```python
from build123d import *

# Parameters (mm, degrees)
EXTRUDE_1_DEPTH     = 24
SKETCH_2_R          = 1.6
CUT_EXTRUDE_1_DEPTH = 6.8
SKETCH_3_R          = 3.15
CUT_EXTRUDE_2_DEPTH = 26.4


with BuildPart() as part:
    # 草圖1 → 填料-伸長1 (new body, symmetric)
    with BuildSketch(Plane.XY):
        Polygon((0, 0), (0, 33), (26.4, 33), (26.4, 0), (22.4, 0), (22.4, 27.2), (4, 27.2), (4, 0), align=None)
    extrude(amount=EXTRUDE_1_DEPTH, both=True)

    # 草圖2 → 除料-伸長1 (cut, through all)
    with BuildSketch(Plane.XZ.offset(-27.2)):
        with Locations((7.719922446, 5.480077554)):
            Circle(SKETCH_2_R)
        with Locations((18.680077554, 5.480077554)):
            Circle(SKETCH_2_R)
        with Locations((18.680077554, -5.480077554)):
            Circle(SKETCH_2_R)
        with Locations((7.719922446, -5.480077554)):
            Circle(SKETCH_2_R)
    extrude(amount=-CUT_EXTRUDE_1_DEPTH, mode=Mode.SUBTRACT)

    # 草圖3 → 除料-伸長2 (cut)
    with BuildSketch(Plane(origin=(26.4, 0, 0), x_dir=(0, 0, -1), z_dir=(1, 0, 0))):
        with Locations((0, 6)):
            Circle(SKETCH_3_R)
        with Locations((15, 6)):
            Circle(SKETCH_3_R)
        with Locations((-15, 6)):
            Circle(SKETCH_3_R)
    extrude(amount=-CUT_EXTRUDE_2_DEPTH, mode=Mode.SUBTRACT)


solid = part.part
```
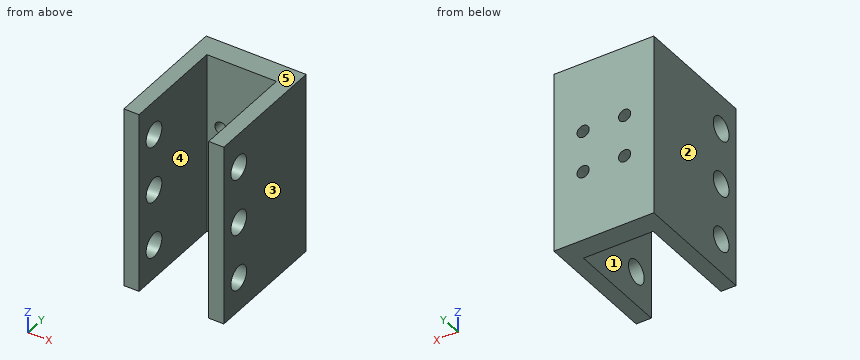
For this review, take the finished solid that the model builds, in its own axes (mm). Face numbers are marked on the shaded views. A direction names the side the tool comes from. Round coordinates to 2 decimals unless told otherwise and drop trailing zeros. Write each loop counter-clockwise with the first axis right and the second up, starting at its lowest first coordinate (ties: lowest second). Pieces come first, ordered by that corner, then holes. Notation, with made-up numbers: M 83.5,55 L 98.5,55 A11 cw 98.5,68 Z; hole C 0.5,-23 d4. An arc over 180 degrees is marked long. One line per item, written item: value. Start each with the question number.
(1) We need section C-C (y = 20.5). Give the boundary of the cut face in (x, z), and give its area (3 significant figures).
(2) We need section B-B (z = 15). Give the boundary of the cut face in (x, y).
(3) We need section D-D (x = 19.5). Give the boundary of the cut face in (y, z), and give its area (3 significant figures).
(4) Insertion check: pin 1 (4 mm diameter, centred on x = 14, z = 16.5, fed in from -Y). The pin has a flat end and moves straight along its axis. Give the tip position at first contact, or say it passes through.
(5) The part is to be moulded in two halves that separate along X. For the marked faces 3, 4 and 5, say which applies: released by +X, released by -X, zero draft, split by the parting line, or undercut.
(6) We need section A-A (y = 6). Count the separate pieces of the cut face and the enclosed holes in it, and give its area (3 significant figures).
(7) Machinability: for the marked faces 1 and 2, which of the approach directions +Z, -Z, +X, -X, +Y, -Y give a long, thin tool a straight path to every point of the face, cutting with its end or side? Answer none if there is none.
(8) Wall thickness on line 1 (X direction, y = 8, z = -7); line 2 (Y direction, x = 22.25, z = 15.5); line 3 (Z direction, x = 24.75, y = 4.5): over which ranges is each line inside the solid? List them lowest first.
Result:
1. outline: M 0,-24 L 4,-24 L 4,24 L 0,24 Z; M 22.4,-24 L 26.4,-24 L 26.4,24 L 22.4,24 Z
1. area: 384 mm²
2. outline: M 0,0 L 4,0 L 4,2.85 L 0,2.85 Z; M 0,9.15 L 4,9.15 L 4,27.2 L 22.4,27.2 L 22.4,9.15 L 26.4,9.15 L 26.4,33 L 0,33 Z; M 22.4,0 L 26.4,0 L 26.4,2.85 L 22.4,2.85 Z
3. outline: M 27.2,-24 L 33,-24 L 33,-6.85 L 27.2,-6.85 Z; M 27.2,-4.11 L 33,-4.11 L 33,4.11 L 27.2,4.11 Z; M 27.2,6.85 L 33,6.85 L 33,24 L 27.2,24 Z
3. area: 247 mm²
4. pin 1: y = 27.2
5. face 3: released by +X
5. face 4: undercut
5. face 5: zero draft
6. separate pieces: 8
6. enclosed holes: 0
6. area: 233 mm²
7. face 1: +Z, -Z, -Y
7. face 2: +Z, -Z, -X, +Y, -Y
8. line 1: 0 to 4, 22.4 to 26.4
8. line 2: 27.2 to 33
8. line 3: -24 to -17.77, -12.23 to -2.77, 2.77 to 12.23, 17.77 to 24
